```python
from build123d import *

# Parameters (mm, degrees)
SKETCH1_W            = 15.5
SKETCH1_H            = 17.5
SKETCH1_W_2          = 5.75
SKETCH1_H_2          = 1
BOSS_EXTRUDE1_DEPTH  = 22.5
CUT_EXTRUDE1_DEPTH   = 2
MIRROR2_COPY_1_DEPTH = 2
SKETCH3_W            = 5.5
SKETCH3_H            = 10.5
CUT_EXTRUDE2_DEPTH   = 10


with BuildPart() as part:
    # Sketch1 → Boss-Extrude1 (new body)
    with BuildSketch(Plane(origin=(0, 0, 0), x_dir=(1, 0, 0), z_dir=(0, 1, 0))):
        Rectangle(SKETCH1_W, SKETCH1_H)
        with Locations((10.625, -8.25)):
            Rectangle(SKETCH1_W_2, SKETCH1_H_2)
        with Locations((-10.625, -8.25)):
            Rectangle(SKETCH1_W_2, SKETCH1_H_2)
    extrude(amount=BOSS_EXTRUDE1_DEPTH)

    # Sketch2 → Cut-Extrude1 (cut, through all)
    with BuildSketch(Plane(origin=(0, 0, 7.75), x_dir=(-1, 0, 0), z_dir=(0, 0, -1))):
        with BuildLine():
            Line((12.375, 18.75), (12.375, 17.25))
            ThreePointArc((12.375, 17.25), (10.625, 15.5), (8.875, 17.25))
            Line((8.875, 17.25), (8.875, 18.75))
            ThreePointArc((8.875, 18.75), (10.625, 20.5), (12.375, 18.75))
        make_face()
    cut_extrude1 = extrude(amount=-CUT_EXTRUDE1_DEPTH, mode=Mode.SUBTRACT)

    # Mirror1: Cut-Extrude1 across plane
    add(cut_extrude1.mirror(Plane(origin=(0, 0, 0), x_dir=(0, 0, 1), z_dir=(1, 0, 0))), mode=Mode.SUBTRACT)

    # Mirror2: Cut-Extrude1 across plane
    add(cut_extrude1.mirror(Plane.ZX.offset(11.25)), mode=Mode.SUBTRACT)

    # Mirror2 copy 1 sketch → Mirror2 copy 1 (cut, through all)
    with BuildSketch(Plane(origin=(0, 22.5, 7.75), x_dir=(1, 0, 0), z_dir=(0, 0, -1))):
        with BuildLine():
            Line((12.375, 18.75), (12.375, 17.25))
            ThreePointArc((12.375, 17.25), (10.625, 15.5), (8.875, 17.25))
            Line((8.875, 17.25), (8.875, 18.75))
            ThreePointArc((8.875, 18.75), (10.625, 20.5), (12.375, 18.75))
        make_face()
    extrude(amount=-MIRROR2_COPY_1_DEPTH, mode=Mode.SUBTRACT)

    # Sketch3 → Cut-Extrude2 (cut)
    with BuildSketch(Plane(origin=(0, 22.5, 0), x_dir=(1, 0, 0), z_dir=(0, 1, 0))):
        Rectangle(SKETCH3_W, SKETCH3_H)
    extrude(amount=-CUT_EXTRUDE2_DEPTH, mode=Mode.SUBTRACT)


solid = part.part
```
Source: CAD feature listing. Evaluate the final solid. Frame: model axes, mm. A direction names the side the tool comes from. Give positions to 0.01 mm unless a question says otherwise; leave off trailing zeros. Order: outer loops, then holes, each group sorted by start corner. A loop starts at its lowest first (then second) coordinate and runs counter-clockwise, first axis right, second up.
(1) Section query C-C (x = 10). Return the cut outline in (y, z), plus the area to 3 significant figures.
(2) Contact query for flat-ended pins moving along their axis: P1, Ø8, axis at y = 6, z = -3, coming from the +X side; P2, Ø1, axis at y = 4.5, z = -3, coming from the -X side. Output: stop coordinate, or through.
(3) Section query D-D (z = -2.75). Return the cut outline in (x, y), plus the area to 3 significant figures.
(4) Material intervals for line 1 along Z through (x, y) = (-1.5, 13.5); line 2 along X through (y, z) = (20.5, -3.5); line 3 along Z through (x, y) = (9, 11.5), sorted ascending.
(5) Access query for faces 1 (the face through (-13.5, 11, 8)), 2 (the face through (-7.75, 11, 0)), 3 (the face through (7.75, 11, 0)), 4 (the face through (2.75, 18, 0)), 5 (the face through (10.7, 15.5, 8.2)). Directions: +Z, -Z, +X, -X, +Y, -Y. A direction counts if a zero-diameter tool reaches every point of the face in a straight line with its end or side. Return the directions, or none.
(6) Section query A-A (y = 4.25). Return the cut outline in (x, z) (3 decimals), plus the area to 3 significant figures.
(7) Section query B-B (y = 18). Return the cut outline in (x, z) (3 decimals), plus the area to 3 significant figures.
(8) Pull-direction query (Y, two-part tool) for faces 6 (the face through (10.6, 2, 8.2)), 7 (the face through (0, 11, -8.75)); classes: +Y half, -Y half, draft (parallel to the pull), parting line (faces both ways), or undercut.
Outcome:
1. outline: (0, 7.75) - (2.12, 7.75) - (2.12, 8.75) - (0, 8.75) - close; (6.88, 7.75) - (15.62, 7.75) - (15.62, 8.75) - (6.88, 8.75) - close; (20.38, 7.75) - (22.5, 7.75) - (22.5, 8.75) - (20.38, 8.75) - close
1. area: 13.0 mm2
2. P1: stops at x = 7.75
2. P2: stops at x = -7.75
3. outline: (-7.75, 0) - (7.75, 0) - (7.75, 22.5) - (2.75, 22.5) - (2.75, 12.5) - (-2.75, 12.5) - (-2.75, 22.5) - (-7.75, 22.5) - close
3. area: 294 mm2
4. line 1: z = -8.75 to -5.25, 5.25 to 8.75
4. line 2: x = -7.75 to -2.75, 2.75 to 7.75
4. line 3: z = 7.75 to 8.75
5. face 1: +Z, -Z, -X, +Y, -Y
5. face 2: -Z, -X, +Y, -Y
5. face 3: -Z, +X, +Y, -Y
5. face 4: +Y
5. face 5: +Z, -Z
6. outline: (-13.5, 7.75) - (-12.375, 7.75) - (-12.375, 8.75) - (-13.5, 8.75) - close; (-8.875, 7.75) - (-7.75, 7.75) - (-7.75, -8.75) - (7.75, -8.75) - (7.75, 7.75) - (8.875, 7.75) - (8.875, 8.75) - (-8.875, 8.75) - close; (12.375, 7.75) - (13.5, 7.75) - (13.5, 8.75) - (12.375, 8.75) - close
6. area: 276 mm2
7. outline: (-13.5, 7.75) - (-12.375, 7.75) - (-12.375, 8.75) - (-13.5, 8.75) - close; (-8.875, 7.75) - (-7.75, 7.75) - (-7.75, -8.75) - (7.75, -8.75) - (7.75, 7.75) - (8.875, 7.75) - (8.875, 8.75) - (-8.875, 8.75) - close; (12.375, 7.75) - (13.5, 7.75) - (13.5, 8.75) - (12.375, 8.75) - close; hole (-2.75, -5.25) - (2.75, -5.25) - (2.75, 5.25) - (-2.75, 5.25) - close
7. area: 218 mm2
8. face 6: undercut
8. face 7: draft
